Build history of the part. All positions in model axes, mm. A direction names the side the tool comes from. Give positions to 0.01 mm unless a question says otherwise; leave off trailing zeros. Write each loop counter-clockwise with the first axis right and the second up, starting at its lowest first coordinate (ties: lowest second). Pieces come first, ordered by that corner, then holes. Notation, with made-up numbers: (18, -5) - (69, -5) arc R31 cw to (69, 32) - close; hole circle Ø10 at (-28, 65). An arc over 180 degrees is marked (long way). Use one line per item in the form item = value. Start each with the question number.
Autodesk Inventor part; units mm, degrees
ref_plane "YZ Plane" through (0, 0, 0) normal (1, 0, 0) x (0, 1, 0)
ref_plane "XZ Plane" through (0, 0, 0) normal (0, 1, 0) x (-1, 0, 0)
ref_plane "XY Plane" through (0, 0, 0) normal (0, 0, 1) x (1, 0, 0)
sketch "Sketch1" plane through (0, 0, 0) normal (1, 0, 0) x (0, 1, 0)
  line L0 (-4.5658, 12.6718) -> (-17.2658, 12.6718)
  line L1 (-23.6158, 6.3218) -> (-23.6158, -82.5782)
  line L2 (-17.2658, -88.9282) -> (-4.5658, -88.9282)
  line L3 (1.7842, -82.5782) -> (1.7842, 6.3218)
  arc A0 (1.7842, 6.3218) -> (-4.5658, 12.6718) centre (-4.5658, 6.3218) ccw
  arc A1 (-17.2658, 12.6718) -> (-23.6158, 6.3218) centre (-17.2658, 6.3218) ccw
  arc A2 (-23.6158, -82.5782) -> (-17.2658, -88.9282) centre (-17.2658, -82.5782) ccw
  arc A3 (-4.5658, -88.9282) -> (1.7842, -82.5782) centre (-4.5658, -82.5782) ccw
  point P0 (0, 0)
  point P1 (1.7842, 12.6718)
  point P2 (-23.6158, -88.9282)
  point P3 (-23.6158, 12.6718)
  point P4 (1.7842, -88.9282)
  dimension "d0" = 25.4
  dimension "d1" = 101.6
  dimension "d4" = 6.35
extrude "Extrusion1" add sketch "Sketch1" along normal blind 4.064
sketch "Sketch2" plane through (4.064, 0, 0) normal (1, 0, 0) x (0, 0, -1)
  arc A0 (82.5782, -23.6158) -> (88.9282, -17.2658) centre (82.5782, -17.2658) ccw
  line L0 (-12.6718, -4.5658) -> (-12.6718, -17.2658)
  line L1 (82.5782, 1.7842) -> (-6.3218, 1.7842)
  line L2 (82.5782, -1.213) -> (-6.3218, -1.213)
  line L3 (-6.3218, -20.6186) -> (82.5782, -20.6186)
  line L4 (-6.3218, -20.6186) -> (82.5782, -20.6186)
  line L5 (82.5782, -20.6186) -> (82.5782, -23.6158)
  line L6 (82.5782, -23.6158) -> (-6.3218, -23.6158)
  line L7 (-6.3218, -23.6158) -> (-6.3218, -20.6186)
  line L8 (-6.3218, -1.213) -> (82.5782, -1.213)
  line L9 (82.5782, -1.213) -> (82.5782, 1.7842)
  line L10 (82.5782, 1.7842) -> (-6.3218, 1.7842)
  line L11 (-6.3218, 1.7842) -> (-6.3218, -1.213)
  point P0 (0, 0)
  dimension "d6" = 19.4056
extrude "Extrusion2" add sketch "Sketch2" along normal blind 25.4
sketch "Sketch3" plane through (4.064, -1.213, 6.3218) normal (0, 0, 1) x (1, 0, 0)
  line L0 (25.4, 2.9972) -> (25.4, 0)
  line L1 (25.4, 2.9972) -> (25.4, 0)
  line L2 (25.4, -19.4056) -> (25.4, -22.4028)
  line L3 (25.4, -22.4028) -> (29.8318, -19.2996)
  line L4 (25.4, -19.4056) -> (25.4, -22.4028)
  line L5 (0, 2.9972) -> (25.4, 2.9972)
  line L6 (25.4, 2.9972) -> (25.4, 0)
  line L7 (25.4, 2.9972) -> (29.8318, -0.106)
  line L8 (29.7989, -0.0829) -> (25.4, 0)
  line L9 (29.8318, -19.2996) -> (25.4, -19.4056)
  point P0 (-4.064, 1.213)
  dimension "d35" = 5.4102
  dimension "d36" = 55
  dimension "d37" = 5.4102
  dimension "d38" = 55
sketch "Sketch4" plane through (0, 0, 0) normal (-1, 0, 0) x (0, 0, 1)
  arc A0 (12.6718, -4.5658) -> (6.3218, 1.7842) centre (6.3218, -4.5658) ccw
  line L0 (-5.4816, 0) -> (-17.3349, 0)
  line L1 (-17.3349, 0) -> (-17.3349, -4.7413)
  line L2 (-17.3349, -4.7413) -> (-5.4816, -4.7413)
  line L3 (-5.4816, -4.7413) -> (-5.4816, 0)
  line L4 (-30.9663, 0) -> (-19.1129, 0)
  line L5 (-19.1129, 0) -> (-19.1129, -4.7413)
  line L6 (-19.1129, -4.7413) -> (-30.9663, -4.7413)
  line L7 (-30.9663, -4.7413) -> (-30.9663, 0)
  line L8 (-32.7443, 0) -> (-44.5976, 0)
  line L9 (-44.5976, -4.7413) -> (-32.7443, -4.7413)
  line L10 (-32.7443, -4.7413) -> (-32.7443, 0)
  line L11 (-44.5976, 0) -> (-44.5976, -4.7413)
  arc A1 (-82.5782, 1.7842) -> (-88.9282, -4.5658) centre (-82.5782, -4.5658) ccw
  line L12 (-58.2289, -4.7413) -> (-58.2289, 0)
  line L13 (-58.2289, 0) -> (-46.3756, 0)
  line L14 (-46.3756, -4.7413) -> (-58.2289, -4.7413)
  line L15 (-46.3756, 0) -> (-46.3756, -4.7413)
  line L16 (-60.0069, 0) -> (-71.8603, 0)
  line L17 (-71.8603, 0) -> (-71.8603, -4.7413)
  line L18 (-71.8603, -4.7413) -> (-60.0069, -4.7413)
  line L19 (-60.0069, -4.7413) -> (-60.0069, 0)
  line L20 (-85.4916, 0) -> (-73.6383, 0)
  line L21 (-73.6383, 0) -> (-73.6383, -4.7413)
  line L22 (-85.4916, -4.7413) -> (-85.4916, 0)
  line L23 (-73.6383, -4.7413) -> (-85.4916, -4.7413)
  line L24 (-3.7036, 0) -> (8.1497, 0)
  line L25 (8.1497, 0) -> (8.1497, -4.7413)
  line L26 (8.1497, -4.7413) -> (-3.7036, -4.7413)
  line L27 (-3.7036, -4.7413) -> (-3.7036, 0)
  point P0 (0, 0)
  dimension "d47" = 1.778
extrude "Extrusion4" add sketch "Sketch4" along normal blind 25.4
extrude "Extrusion6" add sketch "Sketch3" against normal up to surface (88.9 mm away)
sketch "Sketch8" plane through (0, -23.6158, -82.5782) normal (0, -1, 0) x (1, 0, 0)
  point P0 (0, 82.5782)
properties part number "the whole thing"
(1) Two-plate mould, pull along Z, no slides. Class faces 1 (the flat face through (-25.4, -2, -66)), 2 (the flat face through (-13, -2, -17.335)), 3 (the cylindrical face through (2.004, -0.125, 10.861)), 4 (the flat face through (19, 0, -82.578)): +Z half, -Z half, draft (parallel to the pull), parting line (faces both ways), or undercut.
(2) Wall check: line 1 (Y direction, x = 23.5, z = -14.5); line 2 (X direction, y = -10.25, z = -39.5); line 3 (Y direction, x = 30.5, z = -45). Give the ranges that are in metal, low to high. Write a range as from..to.
(3) Pin check, flat tips, straight feed: pin 1 Ø6 at (x, z) = (-14.5, -79.5) entering from -Y; pin 2 Ø4 at (x, y) = (-15, -3.5) entering from -Z; pin 3 Ø2.5 at (x, y) = (-7, -1.5) entering from +Z. Stop position of each tip, or through.
(4) Cut at A-A, the plane x = -7.5. Give the cut face in (y, z).
(5) Which spindle directions (+Z, -Z, +X, -X, +Y, -Y) get a long thin tool onto all of the face, cutting with end or side? Do faces 5 (the flat face through (-13, -4.741, -25)), 6 (the flat face through (-13, -2, -73.638)), 7 (the flat face through (-25.4, -2, -25)), 8 (the flat face through (17, -1.213, -39)), 9 (the flat face through (-13, 0, -52)). Say none if no direction does.
(6) Cut at C-C, the plane z = -52. Give the cut face in (x, y), then the cut area to 3 significant figures.
(7) Cut at B-B, the plane x = 23. Give the cut face in (y, z), then the cut area to 3 significant figures.
Solution:
q1.face_1 = draft
q1.face_2 = undercut
q1.face_3 = +Z half
q1.face_4 = -Z half
q2.line_1 = -23.62..-20.62, -1.21..1.78
q2.line_2 = 0..4.06
q2.line_3 = -22.89..-20.59, -1.23..1.06
q3.pin_1 = -4.74
q3.pin_2 = -85.49
q3.pin_3 = 8.15
q4.outline = (-4.74, -85.49) - (0, -85.49) - (0, -73.64) - (-4.74, -73.64) - close; (-4.74, -71.86) - (0, -71.86) - (0, -60.01) - (-4.74, -60.01) - close; (-4.74, -58.23) - (0, -58.23) - (0, -46.38) - (-4.74, -46.38) - close; (-4.74, -44.6) - (0, -44.6) - (0, -32.74) - (-4.74, -32.74) - close; (-4.74, -30.97) - (0, -30.97) - (0, -19.11) - (-4.74, -19.11) - close; (-4.74, -17.33) - (0, -17.33) - (0, -5.48) - (-4.74, -5.48) - close; (-4.74, -3.7) - (0, -3.7) - (0, 8.15) - (-4.74, 8.15) - close
q5.face_5 = +Z, -Z, -X, -Y
q5.face_6 = -X, +Y, -Y
q5.face_7 = +Z, -Z, -X, +Y, -Y
q5.face_8 = +Z, -Z
q5.face_9 = +Z, -Z, -X, +Y
q6.outline = (-25.4, -4.74) - (0, -4.74) - (0, -23.62) - (29.46, -23.62) - (33.9, -20.51) - (29.46, -20.62) - (4.06, -20.62) - (4.06, -1.21) - (29.46, -1.21) - (33.86, -1.3) - (29.46, 1.78) - (0, 1.78) - (0, 0) - (-25.4, 0) - close
q6.area = 389 mm2
q7.outline = (-23.62, -82.58) - (-20.62, -82.58) - (-20.62, 6.32) - (-23.62, 6.32) - close; (-1.21, -82.58) - (1.78, -82.58) - (1.78, 6.32) - (-1.21, 6.32) - close
q7.area = 533 mm2
